from build123d import *

# Parameters (mm, degrees)
F1_DEPTH = 50
F2_R     = 1


with BuildPart() as f1:
    # F0 (on Front) → F1 (new body)
    with BuildSketch(Plane.XZ):
        Polygon((0, 38), (0, 0), (50, 0), (40, 38), align=None)
    extrude(amount=F1_DEPTH)

    # F2
    f2_edges = [f1.edges().sort_by_distance(p)[0] for p in [
        (40, -25, 38),
        (0, -25, 38),
        (20, 0, 38),
        (20, -50, 38),
        (0, -25, 0),
        (50, -25, 0),
        (25, 0, 0),
        (25, -50, 0),
        (0, -50, 19),
        (45, -50, 19),
        (45, 0, 19),
        (0, 0, 19),
    ]]
    fillet(f2_edges, radius=F2_R)


solid = f1.part
Geometry check sheet. Reference: the model listing, model coordinates, mm. Coordinates: 2 decimals unless noted, no trailing zeros. Order: outer loops, then holes, each group sorted by start corner. A loop starts at its lowest first (then second) coordinate and runs counter-clockwise, first axis right, second up. Notation, with made-up numbers: (-34.75, 83.25) - (1.25, 83.25) arc R36 ccw to (1.25, 121.25) - close; hole circle Ø9 at (55, 39.25). An arc over 180 degrees is marked (long way). Answer in a Markdown table with one row per item. Add a question column.
1) Gauge pin test, flat end, axial feed: P1, Ø10, axis at y = -12, z = 20.5, coming from the +X side. Record the tip position at first contact, or that the pin passes through.
2) Material ranges on line 1 along Y through (x, z) = (43, 25.5); line 2 along X through (y, z) = (-28.5, 36); line 3 along X through (y, z) = (-21.5, 30.5), recorded low to high. Write a range as [from, to].
3) Cross-section at A-A, the plane y = -8. Record the cut outline in (x, z), then the cut area to 3 significant figures.
Check result:
| question | item | result |
|---|---|---|
| 1 | P1 | stops at x = 45.92 |
| 2 | line 1 | y = [-49.69, -0.31] |
| 2 | line 2 | x = [0, 40.53] |
| 2 | line 3 | x = [0, 41.97] |
| 3 | outline | (0, 1) arc R1 ccw to (1, 0) - (48.7, 0) arc R1 ccw to (49.67, 1.25) - (40.2, 37.25) arc R1 ccw to (39.23, 38) - (1, 38) arc R1 ccw to (0, 37) - close |
| 3 | area | 1,710 mm² |
